Drawing for the job (mm, zero at the part's lowest x, y, z). Round coordinates to 2 decimals unless told otherwise and drop trailing zeros. Order: outer loops, then holes, each group sorted by start corner. A loop starts at its lowest first (then second) coordinate and runs counter-clockwise, first axis right, second up. Notation, with made-up numbers: (39, 53.5) -> (91, 53.5) arc R33 cw to (91, 84.5) -> close; hole circle Ø5 at (-3.5, 48.25). An arc over 180 degrees is marked (long way). Use CSV: the item, a comma, the result in double quotes.
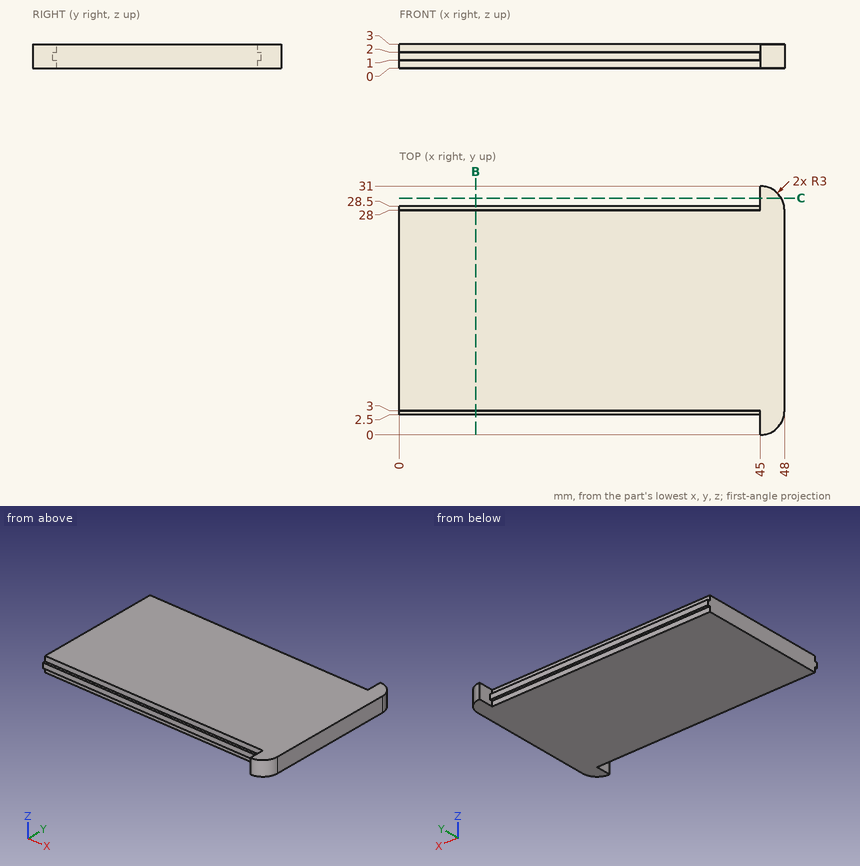
Q1. Probe line 1 along Y through (x, z) = (12.5, 1.2); line 2 along Y through (x, z) = (13, 0.6). List the from-to ranges inside material, lowest first.
From the geometry:
line 1,"y = 2.5 to 28.5"
line 2,"y = 3 to 28"
Q2. Cut at C-C (y = 29.5). Give the cut face in (x, z).
From the geometry:
outline,"(45, 0) -> (47.6, 0) -> (47.6, 3) -> (45, 3) -> close"
Q3. Cut at B-B (x = 9.5). Give the cut face in (y, z).
From the geometry:
outline,"(2.5, 1) -> (3, 1) -> (3, 0) -> (28, 0) -> (28, 1) -> (28.5, 1) -> (28.5, 2) -> (28, 2) -> (28, 3) -> (3, 3) -> (3, 2) -> (2.5, 2) -> close"
Q4. Pin check, flat tips, straight feed: pin 1 (0.8 mm diameter, centred on x = 23.5, z = 2.5, fed in from +Y); pin 2 (1.5 mm diameter, centred on x = 26, y = 6, fed in from -Z); pin 3 (1.1 mm diameter, centred on x = 25, z = 0.5, fed in from -Y); pin 4 (0.5 mm diameter, centred on x = 16, z = 1.5, fed in from +Y). Stop position of each tip, or through.
From the geometry:
pin 1,"stops at y = 28"
pin 2,"stops at z = 0"
pin 3,"stops at y = 2.5"
pin 4,"stops at y = 28.5"
